Part model, mm, in its own coordinate system. A direction names the side the tool comes from. Round coordinates to 2 decimals unless told otherwise and drop trailing zeros. Loops run counter-clockwise (first coordinate to the right, second up) from the corner with the lowest first, then second, coordinate; pieces in that order, holes last. Notation, with made-up numbers: M -18.5,-17.75 L 18.5,-17.75 A27 ccw 18.5,-0.75 Z; hole C -26,14 d2. An arc over 180 degrees is marked long. Write each question's results on one line, items separated by ' | '.
from build123d import *

# Parameters (mm, degrees)
SKETCH_1_W          = 110
SKETCH_1_H          = 20
SKETCH_1_R          = 1.7
EXTRUDE_1_DEPTH     = 4.5
SKETCH_2_W          = 20
SKETCH_2_H          = 8
EXTRUDE_2_DEPTH     = 45
SKETCH_4_W          = 10
SKETCH_4_H          = 10
EXTRUDE_3_DEPTH     = 4.5
SKETCH_5_R          = 1.9
SKETCH_5_R_2        = 1.7
CUT_EXTRUDE_1_DEPTH = 75.885745444
CUT_EXTRUDE_2_DEPTH = 1.3
CUT_EXTRUDE_3_DEPTH = 2.6
SKETCH_7_R          = 1.7
CUT_EXTRUDE_5_DEPTH = 78.673192742
CUT_EXTRUDE_6_DEPTH = 1.3
SKETCH_9_W          = 80
SKETCH_9_H          = 4
EXTRUDE_4_DEPTH     = 50
SKETCH_11_W         = 17.2
SKETCH_11_H         = 50
SKETCH_11_W_2       = 9.3
SKETCH_11_R         = 2.5
SKETCH_11_R_2       = 1.7
CUT_EXTRUDE_7_DEPTH = 90.304255218
RIB_4_REACH         = 124.026
SKETCH_12_WALL_W    = 281.40730074
SKETCH_12_WALL_H    = 3
FILLET_1_R          = 2
FILLET_2_R          = 1.5
FILLET_3_R          = 2
FILLET_4_R          = 12


with BuildPart() as part:
    # 草图1 → 凸台-拉伸1 (new body)
    with BuildSketch(Plane.XY):
        with Locations((0, 10)):
            Rectangle(SKETCH_1_W, SKETCH_1_H)
        with Locations((-45, 14)):
            Circle(SKETCH_1_R, mode=Mode.SUBTRACT)
        with Locations((-30, 14)):
            Circle(SKETCH_1_R, mode=Mode.SUBTRACT)
        with Locations((-15, 14)):
            Circle(SKETCH_1_R, mode=Mode.SUBTRACT)
        with Locations((15, 14)):
            Circle(SKETCH_1_R, mode=Mode.SUBTRACT)
        with Locations((30, 14)):
            Circle(SKETCH_1_R, mode=Mode.SUBTRACT)
        with Locations((45, 14)):
            Circle(SKETCH_1_R, mode=Mode.SUBTRACT)
    extrude(amount=EXTRUDE_1_DEPTH)

    # 草图2 → 凸台-拉伸2 (add)
    with BuildSketch(Plane.XY.offset(4.5)):
        with Locations((-45, 4)):
            Rectangle(SKETCH_2_W, SKETCH_2_H)
        with Locations((45, 4)):
            Rectangle(SKETCH_2_W, SKETCH_2_H)
    extrude(amount=EXTRUDE_2_DEPTH)

    # 草图4 → 凸台-拉伸3 (add)
    with BuildSketch(Plane.XY.offset(4.5)):
        with Locations((-19.238259457, 18.6193749)):
            Rectangle(SKETCH_4_W, SKETCH_4_H)
        with Locations((31.561740543, 18.6193749)):
            Rectangle(SKETCH_4_W, SKETCH_4_H)
    extrude(amount=-EXTRUDE_3_DEPTH)

    # 草图5 → 切除-拉伸1 (cut, through all)
    with BuildSketch(Plane.XY.offset(4.5)):
        with Locations((-19.238259457, 18.6193749)):
            Circle(SKETCH_5_R)
        with Locations((31.561740543, 18.6193749)):
            Circle(SKETCH_5_R)
        with Locations((-15, 14)):
            Circle(SKETCH_5_R_2)
        with Locations((30, 14)):
            Circle(SKETCH_5_R_2)
    extrude(amount=-CUT_EXTRUDE_1_DEPTH, mode=Mode.SUBTRACT)

    # 草图3 → 切除-拉伸2 (cut)
    with BuildSketch(Plane.XY.offset(4.5)):
        Polygon((-45, 17.22), (-47.7886018, 15.61), (-47.7886018, 12.39), (-45, 10.78), (-42.2113982, 12.39), (-42.2113982, 15.61), align=None)
        Polygon((-30, 17.22), (-32.7886018, 15.61), (-32.7886018, 12.39), (-30, 10.78), (-27.2113982, 12.39), (-27.2113982, 15.61), align=None)
        Polygon((-15, 17.22), (-17.7886018, 15.61), (-17.7886018, 12.39), (-15, 10.78), (-12.2113982, 12.39), (-12.2113982, 15.61), align=None)
        Polygon((15, 17.22), (12.2113982, 15.61), (12.2113982, 12.39), (15, 10.78), (17.7886018, 12.39), (17.7886018, 15.61), align=None)
        Polygon((30, 17.22), (27.2113982, 15.61), (27.2113982, 12.39), (30, 10.78), (32.7886018, 12.39), (32.7886018, 15.61), align=None)
        Polygon((45, 17.22), (42.2113982, 15.61), (42.2113982, 12.39), (45, 10.78), (47.7886018, 12.39), (47.7886018, 15.61), align=None)
    extrude(amount=-CUT_EXTRUDE_2_DEPTH, mode=Mode.SUBTRACT)

    # 草图6 → 切除-拉伸3 (cut)
    with BuildSketch(Plane(origin=(0, 0, 0), x_dir=(-1, 0, 0), z_dir=(0, 0, -1))):
        Polygon((-34.861740543, 18.6193749), (-33.211740543, 15.761491068), (-29.911740543, 15.761491068), (-28.261740543, 18.6193749), (-29.911740543, 21.477258733), (-33.211740543, 21.477258733), align=None)
        Polygon((15.938259457, 18.6193749), (17.588259457, 15.761491068), (20.888259457, 15.761491068), (22.538259457, 18.6193749), (20.888259457, 21.477258733), (17.588259457, 21.477258733), align=None)
    extrude(amount=-CUT_EXTRUDE_3_DEPTH, mode=Mode.SUBTRACT)

    # 草图7 → 切除-拉伸5 (cut, through all)
    with BuildSketch(Plane.XZ):
        with Locations(Location((-51, 43.5, 0), (0, 0, 270))):
            Circle(SKETCH_7_R)
        with Locations(Location((-39, 43.5, 0), (0, 0, 270))):
            Circle(SKETCH_7_R)
        with Locations(Location((-45, 33.5, 0), (0, 0, 270))):
            Circle(SKETCH_7_R)
        with Locations(Location((51, 43.5, 0), (0, 0, 270))):
            Circle(SKETCH_7_R)
        with Locations(Location((39, 43.5, 0), (0, 0, 270))):
            Circle(SKETCH_7_R)
        with Locations(Location((45, 33.5, 0), (0, 0, 270))):
            Circle(SKETCH_7_R)
    extrude(amount=-CUT_EXTRUDE_5_DEPTH, mode=Mode.SUBTRACT)

    # 草图8 → 切除-拉伸6 (cut)
    with BuildSketch(Plane(origin=(0, 8, 0), x_dir=(1, 0, 0), z_dir=(0, 1, 0))):
        Polygon((51, -46.72), (53.7886018, -45.11), (53.7886018, -41.89), (51, -40.28), (48.2113982, -41.89), (48.2113982, -45.11), align=None)
        Polygon((39, -46.72), (41.7886018, -45.11), (41.7886018, -41.89), (39, -40.28), (36.2113982, -41.89), (36.2113982, -45.11), align=None)
        Polygon((45, -36.72), (47.7886018, -35.11), (47.7886018, -31.89), (45, -30.28), (42.2113982, -31.89), (42.2113982, -35.11), align=None)
        Polygon((-39, -46.72), (-36.2113982, -45.11), (-36.2113982, -41.89), (-39, -40.28), (-41.7886018, -41.89), (-41.7886018, -45.11), align=None)
        Polygon((-51, -46.72), (-48.2113982, -45.11), (-48.2113982, -41.89), (-51, -40.28), (-53.7886018, -41.89), (-53.7886018, -45.11), align=None)
        Polygon((-45, -36.72), (-42.2113982, -35.11), (-42.2113982, -31.89), (-45, -30.28), (-47.7886018, -31.89), (-47.7886018, -35.11), align=None)
    extrude(amount=-CUT_EXTRUDE_6_DEPTH, mode=Mode.SUBTRACT)

    # 草图9 → 凸台-拉伸4 (add)
    with BuildSketch(Plane.XZ):
        with Locations((-14, 2)):
            Rectangle(SKETCH_9_W, SKETCH_9_H)
    extrude(amount=EXTRUDE_4_DEPTH)

    # 草图11 → 切除-拉伸7 (cut, through all)
    with BuildSketch(Plane(origin=(0, 0, 0), x_dir=(-1, 0, 0), z_dir=(0, 0, -1))):
        with Locations((-17.4, -25)):
            Rectangle(SKETCH_11_W, SKETCH_11_H)
        with Locations((49.35, -25)):
            Rectangle(SKETCH_11_W_2, SKETCH_11_H)
        with Locations((21.7, -46.25)):
            Circle(SKETCH_11_R)
        with Locations((14.7, -46.25)):
            Circle(SKETCH_11_R_2)
        with Locations((28.7, -46.25)):
            Circle(SKETCH_11_R_2)
        with Locations((21.7, -39.25)):
            Circle(SKETCH_11_R_2)
        with Locations((21.7, -32.25)):
            Circle(SKETCH_11_R_2)
        with Locations((14.7, -25.25)):
            Circle(SKETCH_11_R_2)
        with Locations((21.7, -18.25)):
            Circle(SKETCH_11_R_2)
        with Locations((28.7, -25.25)):
            Circle(SKETCH_11_R_2)
        with Locations((21.7, -25.25)):
            Circle(SKETCH_11_R)
        with Locations((4.2, -35.75)):
            Circle(SKETCH_11_R_2)
    extrude(amount=-CUT_EXTRUDE_7_DEPTH, mode=Mode.SUBTRACT)

    # 草图12 wall → 筋4 (add, up to next)
    with BuildSketch(Plane(origin=(-44.7, -12.5, 16.5), x_dir=(0, 0.707106781187, 0.707106781187), z_dir=(0, 0.707106781187, -0.707106781187)), mode=Mode.PRIVATE) as rib_4_sk1:
        with Locations((0, 1.5)):
            Rectangle(SKETCH_12_WALL_W, SKETCH_12_WALL_H)
    rib_4_tool1 = extrude(rib_4_sk1.sketch, amount=RIB_4_REACH, mode=Mode.PRIVATE) - part.part
    add(rib_4_tool1.solids().sort_by_distance((-44.7, -12.5, 16.5))[0])

    # 圆角1
    fillet_1_edges = [part.edges().sort_by_distance(p)[0] for p in [
        (-35, 4, 4.5),
        (-45, 8, 4.5),
        (45, 8, 4.5),
        (35, 4, 4.5),
        (-44.7, 0, 14.5),
        (-41.7, -12.5, 4),
        (-41.7, 0, 16.5),
    ]]
    fillet(fillet_1_edges, radius=FILLET_1_R)

    # 圆角2
    fillet_2_edges = [part.edges().sort_by_distance(p)[0] for p in [
        (-44.7, -50, 2),
        (8.8, -50, 2),
        (-24.238259457, 20, 2.25),
        (-14.238259457, 23.6193749, 2.25),
        (-14.238259457, 20, 2.25),
        (-24.238259457, 23.6193749, 2.25),
        (-55, 20, 2.25),
        (55, 20, 2.25),
        (36.561740543, 23.6193749, 2.25),
        (36.561740543, 20, 2.25),
        (26.561740543, 20, 2.25),
        (26.561740543, 23.6193749, 2.25),
    ]]
    fillet(fillet_2_edges, radius=FILLET_2_R)

    # 圆角3
    fillet_3_edges = [part.edges().sort_by_distance(p)[0] for p in [
        (-55, 4, 49.5),
        (-35, 4, 49.5),
        (55, 4, 49.5),
        (35, 4, 49.5),
    ]]
    fillet(fillet_3_edges, radius=FILLET_3_R)

    # 圆角4
    fillet_4_edges = [part.edges().sort_by_distance(p)[0] for p in [
        (8.8, 0, 2),
    ]]
    fillet(fillet_4_edges, radius=FILLET_4_R)


solid = part.part
Item 1: Band-saw the part on D-D on y = -46.25. Give the cut face in (x, z), and give its area (3 significant figures).
Filled sheet:
outline: M -44.7,0 L -30.4,0 L -30.4,4 L -44.7,4 Z; M -27,0 L -24.2,0 L -24.2,4 L -27,4 Z; M -19.2,0 L -16.4,0 L -16.4,4 L -19.2,4 Z; M -13,0 L 8.8,0 L 8.8,4 L -13,4 Z | area: 167 mm^2
Item 2: Drop flat-ended pins along their axis: P1, Ø16, axis at x = -48, z = 38, coming from the +Y side; P2, Ø10, axis at x = -26, y = 4.5, coming from the -Z side; P3, Ø1.5, axis at y = -12, z = 6, coming from the -X side; P4, Ø0.7, axis at y = 22, z = 1.5, coming from the +X side. Give the stop position or say it passes through.
Filled sheet:
P1: y = 8 | P2: z = 0 | P3: x = -44.7 | P4: x = 36.56
Item 3: Which spindle directions (+Z, -Z, +X, -X, +Y, -Y) get a long thin tool onto all of the face, cutting with end or side? Do faces 1 (the flat face through (-45, 8, 28)), 2 (the flat face through (-52.3, 6.7, 44.9)), 3 (the flat face through (28.7, 12.6, 3.2)), 4 (the flat face through (30, 20, 2.6)). Say none if no direction does.
Filled sheet:
face 1: +Z, +X, -X, +Y | face 2: +Y | face 3: +Z | face 4: -Z
Item 4: Wall check: L1, parallel to X at y = 1.5, z = 10.5; L2, parallel to X at y = 1, z = 5.5; L3, parallel to X at y = 3, z = 43. Give the ranges that are in metal, low to high.
Filled sheet:
L1: -55 to -35, 35 to 55 | L2: -55 to -34.73, 34.73 to 55 | L3: -55 to -52.62, -49.38 to -40.62, -37.38 to -35, 35 to 37.38, 40.62 to 49.38, 52.62 to 55
Item 5: Band-saw the part on B-B on z = 12. Give the cut face in (x, y).
Filled sheet:
outline: M -55,0 L -46.7,0 A2 cw -44.7,-2 L -44.7,-17 L -41.7,-17 L -41.7,-2 A2 cw -39.7,0 L -35,0 L -35,8 L -55,8 Z; M 35,0 L 55,0 L 55,8 L 35,8 Z
Item 6: Band-saw the part on C-C on x = -4.2. Give the cut face in (y, z).
Filled sheet:
outline: M -50,0 L -37.45,0 L -37.45,4 L -50,4 Z; M -34.05,0 L 20,0 L 20,4.5 L 0,4.5 L 0,4 L -34.05,4 Z
Item 7: Band-saw the part on A-A on y = -35.75. Give the cut face in (x, z), and give its area (3 significant figures).
Filled sheet:
outline: M -44.7,0 L -5.9,0 L -5.9,4 L -44.7,4 Z; M -2.5,0 L 8.8,0 L 8.8,4 L -2.5,4 Z | area: 200 mm^2
Item 8: Two-plate mould, pull along Y, no slides. Class faces 5 (the cylindrical face through (12.41, -3.42, 2.03)), 6 (the cylindrical face through (-21.2, -48.7, 2)), 7 (the flat face through (45, 8, 28)): +Y half, -Y half, draft (parallel to the pull), parting line (faces both ways), or undercut.
Filled sheet:
face 5: -Y half | face 6: undercut | face 7: +Y half
